Design review of the part built by this model. Coordinates are the model's own, in mm. A direction names the side the tool comes from. Round coordinates to 2 decimals unless told otherwise and drop trailing zeros. Order: outer loops, then holes, each group sorted by start corner. A loop starts at its lowest first (then second) coordinate and runs counter-clockwise, first axis right, second up. Notation, with made-up numbers: M 1,68.25 L 28,68.25 A22 cw 28,84.25 Z; hole C -7.5,-2.5 d7. An arc over 180 degrees is marked long. Use a Markdown table: item, result. Add a question column.
(1) Take a section at B-B (z = 16). Write out the cut boundary in (x, y), then the cut area to 3 significant figures.
(2) Take a section at C-C (y = 0.5). Write out the cut boundary in (x, z), then the cut area to 3 significant figures.
(3) For pin 1 (1 mm diameter, centred on y = 2, z = 6.5, fed in from -X); pin 2 (1.8 mm diameter, centred on x = -10.5, y = 8.5, fed in from +Z); pin 3 (8 mm diameter, centred on x = 10, y = 7.5, fed in from +Z); pin 4 (2.5 mm diameter, centred on y = 8.5, z = 16, fed in from -X), all flat-tipped, find the tip position at first contact; note any pin that passes through.
(4) Take a section at D-D (x = 2.5). Write out the cut boundary in (y, z).
(5) The part is to be moulded in two halves that separate along Z. For faces 1 (the face through (-12.21, -5.47, 3.32)), 2 (the face through (0, 0, 0)), 3 (the face through (0.07, -8.004, 14.426)), say which applies: released by +Z, released by -Z, zero draft, split by the parting line, or undercut.
(6) Take a section at A-A (x = -10). Write out the cut boundary in (y, z), then the cut area to 3 significant figures.
(7) Machinability: for faces 4 (the face through (9, 0, 5)), 5 (the face through (-0.1, -11, 18.5)), 6 (the face through (-8, 8, 1.6)), which of the approach directions +Z, -Z, +X, -X, +Y, -Y give a long, thin tool a straight path to every point of the face, cutting with its end or side? Answer none if there is none.
(8) To check wall thickness, follow probe 1 along Y at (x, z) = (10, 0.75); probe 2 along Y at (x, z) = (-2.5, 16); probe 3 along Z at (x, y) = (-10.25, 1.5). State the ranges of each line that lie inside material, in increasing order. Write a range as from..to.
```python
from build123d import *

# Parameters (mm, degrees)
SKETCH1_W                                            = 27
SKETCH1_H                                            = 25
BOSS_EXTRUDE1_DEPTH                                  = 5
SKETCH2_W                                            = 10
SKETCH2_H                                            = 25
BOSS_EXTRUDE2_DEPTH                                  = 15
CBORE_FOR_M3_HEXAGON_SOCKET_HEAD_CAP_SCR_D           = 3.4
CBORE_FOR_M3_HEXAGON_SOCKET_HEAD_CAP_SCR_CBORE_D     = 6
CBORE_FOR_M3_HEXAGON_SOCKET_HEAD_CAP_SCR_CBORE_DEPTH = 3.4
M4_TAPPED_HOLE1_D                                    = 3.3
CHAMFER1_SIZE                                        = 3


with BuildPart() as part:
    # Sketch1 → Boss-Extrude1 (new body)
    with BuildSketch(Plane.XY):
        Rectangle(SKETCH1_W, SKETCH1_H)
    extrude(amount=BOSS_EXTRUDE1_DEPTH)

    # Sketch2 → Boss-Extrude2 (add)
    with BuildSketch(Plane.XY.offset(5)):
        Rectangle(SKETCH2_W, SKETCH2_H)
    extrude(amount=BOSS_EXTRUDE2_DEPTH)

    # CBORE for M3 Hexagon socket head cap screws1 (through all)
    with Locations(Plane.XY.offset(5)):
        with Locations((10, 7.5), (10, -7.5), (-10, -7.5), (-10, 7.5)):
            CounterBoreHole(CBORE_FOR_M3_HEXAGON_SOCKET_HEAD_CAP_SCR_D / 2, CBORE_FOR_M3_HEXAGON_SOCKET_HEAD_CAP_SCR_CBORE_D / 2, CBORE_FOR_M3_HEXAGON_SOCKET_HEAD_CAP_SCR_CBORE_DEPTH)

    # M4 Tapped Hole1 (through all)
    with Locations(Plane.ZY.offset(5)):
        with Locations((16, 8.5), (16, -8.5)):
            Hole(M4_TAPPED_HOLE1_D / 2)

    # Chamfer1
    chamfer1_edges = [part.edges().sort_by_distance(p)[0] for p in [
        (0, 12.5, 20),
        (0, -12.5, 20),
        (13.5, -12.5, 2.5),
        (-13.5, -12.5, 2.5),
        (-13.5, 12.5, 2.5),
        (13.5, 12.5, 2.5),
    ]]
    chamfer(chamfer1_edges, length=CHAMFER1_SIZE)


solid = part.part
```
Verdict:
| question | item | result |
|---|---|---|
| 1 | outline | M -5,-12.5 L 5,-12.5 L 5,-10.15 L -5,-10.15 Z; M -5,-6.85 L 5,-6.85 L 5,6.85 L -5,6.85 Z; M -5,10.15 L 5,10.15 L 5,12.5 L -5,12.5 Z |
| 1 | area | 184 mm^2 |
| 2 | outline | M -13.5,0 L 13.5,0 L 13.5,5 L 5,5 L 5,20 L -5,20 L -5,5 L -13.5,5 Z |
| 2 | area | 285 mm^2 |
| 3 | pin 1 | stops at x = -5 |
| 3 | pin 2 | stops at z = 1.6 |
| 3 | pin 3 | stops at z = 5 |
| 3 | pin 4 | passes through |
| 4 | outline | M -12.5,0 L 12.5,0 L 12.5,17 L 9.5,20 L -9.5,20 L -12.5,17 Z; hole C -8.5,16 d3.3; hole C 8.5,16 d3.3 |
| 5 | face 1 | zero draft |
| 5 | face 2 | released by -Z |
| 5 | face 3 | undercut |
| 6 | outline | M -12.5,0 L -9.2,0 L -9.2,1.6 L -10.5,1.6 L -10.5,5 L -12.5,5 Z; M -5.8,0 L 5.8,0 L 5.8,1.6 L 4.5,1.6 L 4.5,5 L -4.5,5 L -4.5,1.6 L -5.8,1.6 Z; M 9.2,0 L 12.5,0 L 12.5,5 L 10.5,5 L 10.5,1.6 L 9.2,1.6 Z |
| 6 | area | 73.3 mm^2 |
| 7 | face 4 | +Z, +X, +Y, -Y |
| 7 | face 5 | +Z, +X, -X, -Y |
| 7 | face 6 | +Z |
| 8 | probe 1 | y = -12.5..-9.2, -5.8..5.8, 9.2..12.5 |
| 8 | probe 2 | y = -12.5..-10.15, -6.85..6.85, 10.15..12.5 |
| 8 | probe 3 | z = 0..5 |
